```python
from build123d import *

# Parameters (mm, degrees)
SKETCH1_R           = 12.7
BOSS_EXTRUDE1_DEPTH = 23.75
FILLET1_R           = 10
SKETCH2_R           = 2.9
BOSS_EXTRUDE2_DEPTH = 5


with BuildPart() as part:
    # Sketch1 → Boss-Extrude1 (new body)
    with BuildSketch(Plane(origin=(0, 0, 0), x_dir=(1, 0, 0), z_dir=(0, 1, 0))):
        with Locations(Location((0, 0, 0), (0, 0, 270))):
            Circle(SKETCH1_R)
    extrude(amount=BOSS_EXTRUDE1_DEPTH)

    # Fillet1
    fillet1_edges = [part.edges().sort_by_distance(p)[0] for p in [
        (0, 23.75, -12.7),
    ]]
    fillet(fillet1_edges, radius=FILLET1_R)

    # Sketch2 → Boss-Extrude2 (add)
    with BuildSketch(Plane.XZ):
        with BuildLine():
            Line((7.5, 19), (7.5, -19))
            ThreePointArc((7.5, -19), (0, -26.5), (-7.5, -19))
            Line((-7.5, -19), (-7.5, 19))
            ThreePointArc((-7.5, 19), (0, 26.5), (7.5, 19))
        make_face()
        with Locations(Location((0, 19, 0), (0, 0, 270))):
            Circle(SKETCH2_R, mode=Mode.SUBTRACT)
        with Locations(Location((0, -19, 0), (0, 0, 270))):
            Circle(SKETCH2_R, mode=Mode.SUBTRACT)
    extrude(amount=-BOSS_EXTRUDE2_DEPTH)


solid = part.part
```
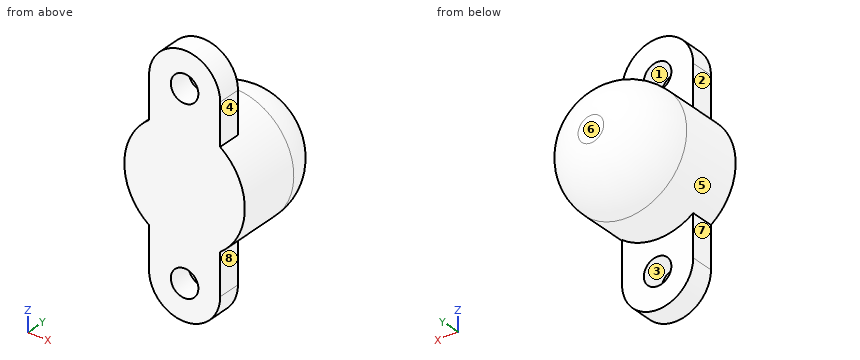
Can you work these out from the model? Positions are in its coordinate system, mm. Face numbers are marked on the shaded views. A direction names the side the tool comes from. Give positions to 0.01 mm unless a question says otherwise; leave off trailing zeros. Order: outer loops, then holes, each group sorted by start corner. A loop starts at its lowest first (then second) coordinate and runs counter-clockwise, first axis right, second up. Notation, with made-up numbers: (-14, -4.75) - (19, -4.75) arc R32 ccw to (19, 27.25) - close; hole circle Ø3 at (-29, -3.5). An arc over 180 degrees is marked (long way). Use a Markdown table: item, result. Add a question column.
Q1. If we mould it in two halves opening along X, with no side actions, what happens to the marked faces 1, 2, 3 and 4? For each: released by +X, released by -X, zero draft, split by the parting line, or undercut.
Q2. If we section it at C-C on z = 14: Write out the boundary of the cut face in (x, y), plus the area to 3 significant figures.
Q3. On a 3-axis mill with a long thin cutter (end or side, diameter ignored), from which of +Z, -Z, +X, -X, +Y, -Y can I reach the whole of each face in a straight line? I mean the marked faces 5, 6, 7 and 8. Say none if no direction works.
Q4. If we section it at A-A on z = -20.5: Write out the boundary of the cut face in (x, y).
Q5. If we section it at D-D on z = 20: Write out the boundary of the cut face in (x, y).
Q6. I'm going to push flat-ended pins straight in: pin 1 (6 mm diameter, centred on y = 7, z = -13, fed in from -X); pin 2 (6.5 mm diameter, centred on x = 0, z = 19, fed in from +Y); pin 3 (8 mm diameter, centred on x = 5, y = 4.5, fed in from -Z). Where does each tip first touch, or does it pass through?
Q7. Please list where these lines run through material, in increasing order: line 1 along X through (y, z) = (2.5, -19); line 2 along Y through (x, z) = (3, 13.5); line 3 along X through (y, z) = (1.5, -15).
Q8. If we section it at B-B on x = 0: Count the separate pieces of the cut face and the enclosed holes in it, plus the area to 3 significant figures.
Answers follow:
| question | item | result |
|---|---|---|
| 1 | face 1 | undercut |
| 1 | face 2 | released by -X |
| 1 | face 3 | undercut |
| 1 | face 4 | released by +X |
| 2 | outline | (-7.5, 0) - (7.5, 0) - (7.5, 5) - (-7.5, 5) - close |
| 2 | area | 75.0 mm^2 |
| 3 | face 5 | +Y |
| 3 | face 6 | +Z, -Z, +X, -X, +Y |
| 3 | face 7 | -Z, -X, +Y, -Y |
| 3 | face 8 | -Z, +X, +Y, -Y |
| 4 | outline | (-7.35, 0) - (-2.48, 0) - (-2.48, 5) - (-7.35, 5) - close; (2.48, 0) - (7.35, 0) - (7.35, 5) - (2.48, 5) - close |
| 5 | outline | (-7.43, 0) - (-2.72, 0) - (-2.72, 5) - (-7.43, 5) - close; (2.72, 0) - (7.43, 0) - (7.43, 5) - (2.72, 5) - close |
| 6 | pin 1 | stops at x = -7.83 |
| 6 | pin 2 | stops at y = 5 |
| 6 | pin 3 | stops at z = -26.43 |
| 7 | line 1 | x = -7.5 to -2.9, 2.9 to 7.5 |
| 7 | line 2 | y = 0 to 5 |
| 7 | line 3 | x = -7.5 to 7.5 |
| 8 | separate pieces | 3 |
| 8 | enclosed holes | 0 |
| 8 | area | 640 mm^2 |
